from build123d import *

# Parameters (mm, degrees)
SKETCH_1_R          = 10
EXTRUDE_1_DEPTH     = 3
SKETCH_2_R          = 0.75
CUT_EXTRUDE_1_DEPTH = 15.456832295
SKETCH_3_R          = 5
EXTRUDE_2_DEPTH     = 19.4
SKETCH_6_W          = 19.4
SKETCH_6_H          = 5
EXTRUDE_4_DEPTH     = 53
CUT_EXTRUDE_2_DEPTH = 58.742788457
SKETCH_8_R          = 1.5
CUT_EXTRUDE_3_DEPTH = 59.401712304
FILLET_1_R          = 2


with BuildPart() as part:
    # 草图1 → 凸台-拉伸1 (new body)
    with BuildSketch(Plane.XY):
        Circle(SKETCH_1_R)
    extrude(amount=EXTRUDE_1_DEPTH)

    # 草图2 → 切除-拉伸1 (cut, through all)
    with BuildSketch(Plane(origin=(0, 0, 0), x_dir=(-1, 0, 0), z_dir=(0, 0, -1))):
        with Locations((0, 7)):
            Circle(SKETCH_2_R)
        with Locations((7, 0)):
            Circle(SKETCH_2_R)
        with Locations((0, -7)):
            Circle(SKETCH_2_R)
        with Locations((-7, 0)):
            Circle(SKETCH_2_R)
    extrude(amount=-CUT_EXTRUDE_1_DEPTH, mode=Mode.SUBTRACT)

    # 草图3 → 凸台-拉伸2 (add)
    with BuildSketch(Plane(origin=(0, 0, 0), x_dir=(-1, 0, 0), z_dir=(0, 0, -1))):
        with Locations(Location((0, 0, 0), (0, 0, 180))):
            Circle(SKETCH_3_R)
    extrude(amount=EXTRUDE_2_DEPTH)

    # 草图6 → 凸台-拉伸4 (add)
    with BuildSketch(Plane(origin=(0, 0, 0), x_dir=(0, 0, -1), z_dir=(1, 0, 0))):
        with Locations((9.7, 0.298786174)):
            Rectangle(SKETCH_6_W, SKETCH_6_H)
    extrude(amount=EXTRUDE_4_DEPTH)

    # 草图7 → 切除-拉伸2 (cut, through all)
    with BuildSketch(Plane(origin=(0, -2.201213826, 0), x_dir=(-1, 0, 0), z_dir=(0, -1, 0))):
        with BuildLine():
            Line((-4.489393911, -0.038773437), (-53, -0.038773437))
            Line((-53, -0.038773437), (-53, 14.4))
            Line((-53, 14.4), (-10.989393911, 14.4))
            ThreePointArc((-10.989393911, 14.4), (-6.393199834, 12.496194078), (-4.489393911, 7.9))
            Line((-4.489393911, 7.9), (-4.489393911, -0.038773437))
        make_face()
    extrude(amount=-CUT_EXTRUDE_2_DEPTH, mode=Mode.SUBTRACT)

    # 草图8 → 切除-拉伸3 (cut, through all)
    with BuildSketch(Plane(origin=(0, 0, -19.4), x_dir=(-1, 0, 0), z_dir=(0, 0, -1))):
        with Locations((-46, 0.261084443)):
            Circle(SKETCH_8_R)
    extrude(amount=-CUT_EXTRUDE_3_DEPTH, mode=Mode.SUBTRACT)

    # 圆角1
    fillet_1_edges = [part.edges().sort_by_distance(p)[0] for p in [
        (53, 2.798786174, -16.9),
        (53, -2.201213826, -16.9),
    ]]
    fillet(fillet_1_edges, radius=FILLET_1_R)


solid = part.part
Could you check a few things on this model? Use its own coordinates, in mm. A direction names the side the tool comes from. Round coordinates to 2 decimals unless told otherwise and drop trailing zeros. Loops run counter-clockwise (first coordinate to the right, second up) from the corner with the lowest first, then second, coordinate; pieces in that order, holes last. Notation, with made-up numbers: (44.25, 21) - (101.25, 21) arc R14 cw to (101.25, 44) - close; hole circle Ø2 at (40, 39.25). An arc over 180 degrees is marked (long way). Write item = value, one per line.
1) Imagine slicing it at B-B (x = 46). Please give me the cut outline in (y, z), and give its area (4 significant figures).
Computed:
outline = (-2.2, -19.4) - (-1.24, -19.4) - (-1.24, -14.4) - (-2.2, -14.4) - close; (1.76, -19.4) - (2.8, -19.4) - (2.8, -14.4) - (1.76, -14.4) - close
area = 10.00 mm2
2) I'm going to push flat-ended pins straight in: P1, Ø1.4, axis at x = 0, y = 7, coming from the -Z side (3 decimals); P2, Ø1.7, axis at x = 0, y = -7, coming from the -Z side; P3, Ø2.5, axis at x = 32, y = 1.5, coming from the +Z side; P4, Ø3, axis at y = 6, z = -12, coming from the +X side. Where does each tip first touch, or does it pass through?
Computed:
P1 = through
P2 = 0
P3 = -14.4
P4 = 2.18
3) On a 3-axis mill with a long thin cutter (end or side, diameter ignored), from which of +Z, -Z, +X, -X, +Y, -Y can I reach the whole of each face in a straight line? I mean faces 1 (the cylindrical face through (-4.97, -0.53, -9.56)), 2 (the flat face through (26, 2.799, -17)), 3 (the flat face through (27, -2.201, -16)). Say none if no direction works.
Computed:
face_1 = -Z
face_2 = -Z, +X, +Y
face_3 = -Z, +X, -Y
4) Imagine slicing it at D-D (z = -15). Please give me the cut outline in (x, y).
Computed:
outline = (4.14, 2.8) arc R5 ccw (long way) to (4.49, -2.2) - (51, -2.2) arc R2 ccw to (53, -0.2) - (53, 0.8) arc R2 ccw to (51, 2.8) - close; hole circle Ø3 at (46, 0.26)
5) I need wall thicknesses on line 1 along Y through (x, z) = (0, 1.9); line 2 along Y through (x, z) = (46, -15.65); line 3 along Z through (x, y) = (35.5, 1.75). Which ranges of each line are inside material? Lowest first, please. Write a range as from..to.
Computed:
line_1 = -10..-7.75, -6.25..6.25, 7.75..10
line_2 = -2.2..-1.24, 1.76..2.8
line_3 = -19.4..-14.4
6) Imagine slicing it at C-C (y = -7). Please give me the cut outline in (x, z), and give its area (3 significant figures).
Computed:
outline = (-7.14, 0) - (-0.75, 0) - (-0.75, 3) - (-7.14, 3) - close; (0.75, 0) - (7.14, 0) - (7.14, 3) - (0.75, 3) - close
area = 38.3 mm2
7) Imagine slicing it at A-A (x = 0). Please give me the cut outline in (y, z).
Computed:
outline = (-10, 0) - (-7.75, 0) - (-7.75, 3) - (-10, 3) - close; (-6.25, 0) - (-5, 0) - (-5, -19.4) - (5, -19.4) - (5, 0) - (6.25, 0) - (6.25, 3) - (-6.25, 3) - close; (7.75, 0) - (10, 0) - (10, 3) - (7.75, 3) - close
8) If we mould it in two halves opening along Z, with no side actions, what happens to faces 4 (the flat face through (-5, -2, 0)), 5 (the cylindrical face through (47.5, 0.3, -16.9)), 6 (the flat face through (7, 2, 0.039))? For each: pulls with the +Z half, pulls with the -Z half, needs draft (parallel to the pull), parting line crosses it, or undercut.
Computed:
face_4 = pulls with the -Z half
face_5 = needs draft
face_6 = undercut
